CAD build for the part. Positions are in the model's coordinates, mm. Round coordinates to 2 decimals unless told otherwise and drop trailing zeros. Order: outer loops, then holes, each group sorted by start corner. A loop starts at its lowest first (then second) coordinate and runs counter-clockwise, first axis right, second up. Notation, with made-up numbers: M 88.25,77 L 138.25,77 A16 cw 138.25,96 Z; hole C 87,-22 d3. An arc over 180 degrees is marked long. Put each result on its own line as item: value.
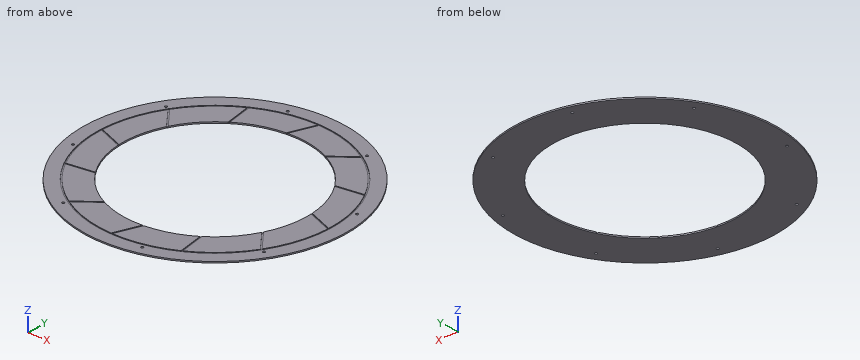
```python
from build123d import *

# Parameters (mm, degrees)
SKETCH1_R                    = 254
SKETCH1_R_2                  = 177.8
BOSS_EXTRUDE1_DEPTH          = 2.54
SKETCH2_R                    = 228.6
SKETCH2_R_2                  = 226.06
CUT_EXTRUDE1_DEPTH           = 1.27
CUT_EXTRUDE2_DEPTH           = 1.27
F_10_0_1935_DIAMETER_HOLE2_D = 4.9149


with BuildPart() as part:
    # Sketch1 → Boss-Extrude1 (new body)
    with BuildSketch(Plane.XY):
        Circle(SKETCH1_R)
        Circle(SKETCH1_R_2, mode=Mode.SUBTRACT)
    extrude(amount=BOSS_EXTRUDE1_DEPTH)

    # Sketch2 → Cut-Extrude1 (cut)
    with BuildSketch(Plane.XY.offset(2.54)):
        Circle(SKETCH2_R)
        Circle(SKETCH2_R_2, mode=Mode.SUBTRACT)
    extrude(amount=-CUT_EXTRUDE1_DEPTH, mode=Mode.SUBTRACT)

    # Sketch4 → Cut-Extrude2 (cut)
    with BuildSketch(Plane.XY.offset(2.54)):
        with BuildLine():
            Line((-226.06, 0), (-176.125415463, -18.479751401))
            Line((-176.125415463, -18.479751401), (-175.243846947, -16.097643731))
            Line((-175.243846947, -16.097643731), (-226.043846947, 2.702379938))
            ThreePointArc((-226.043846947, 2.702379938), (-226.055961701, 1.351214107), (-226.06, 0))
        make_face()
        with BuildLine():
            Line((-195.77370278, 113.03), (-161.768959743, 72.058773562))
            Line((-161.768959743, 72.058773562), (-159.814445179, 73.680955061))
            Line((-159.814445179, 73.680955061), (-194.408523857, 115.36225315))
            ThreePointArc((-194.408523857, 115.36225315), (-195.094598456, 114.198166593), (-195.77370278, 113.03))
        make_face()
        with BuildLine():
            Line((-113.03, 195.77370278), (-104.066641901, 143.289208342))
            Line((-104.066641901, 143.289208342), (-101.562891886, 143.716801448))
            Line((-101.562891886, 143.716801448), (-110.681593797, 197.110903794))
            ThreePointArc((-110.681593797, 197.110903794), (-111.857795108, 196.445812563), (-113.03, 195.77370278))
        make_face()
        with BuildLine():
            Line((0, 226.06), (-18.479751401, 176.125415463))
            Line((-18.479751401, 176.125415463), (-16.097643731, 175.243846947))
            Line((-16.097643731, 175.243846947), (2.702379938, 226.043846947))
            ThreePointArc((2.702379938, 226.043846947), (1.351214107, 226.055961701), (0, 226.06))
        make_face()
        with BuildLine():
            Line((113.03, 195.77370278), (72.058773562, 161.768959743))
            Line((72.058773562, 161.768959743), (73.680955061, 159.814445179))
            Line((73.680955061, 159.814445179), (115.36225315, 194.408523857))
            ThreePointArc((115.36225315, 194.408523857), (114.198166593, 195.094598456), (113.03, 195.77370278))
        make_face()
        with BuildLine():
            Line((195.77370278, 113.03), (143.289208342, 104.066641901))
            Line((143.289208342, 104.066641901), (143.716801448, 101.562891886))
            Line((143.716801448, 101.562891886), (197.110903794, 110.681593797))
            ThreePointArc((197.110903794, 110.681593797), (196.445812563, 111.857795108), (195.77370278, 113.03))
        make_face()
        with BuildLine():
            Line((226.06, 0), (176.125415463, 18.479751401))
            Line((176.125415463, 18.479751401), (175.243846947, 16.097643731))
            Line((175.243846947, 16.097643731), (226.043846947, -2.702379938))
            ThreePointArc((226.043846947, -2.702379938), (226.055961701, -1.351214107), (226.06, 0))
        make_face()
        with BuildLine():
            Line((195.77370278, -113.03), (161.768959743, -72.058773562))
            Line((161.768959743, -72.058773562), (159.814445179, -73.680955061))
            Line((159.814445179, -73.680955061), (194.408523857, -115.36225315))
            ThreePointArc((194.408523857, -115.36225315), (195.094598456, -114.198166593), (195.77370278, -113.03))
        make_face()
        with BuildLine():
            Line((113.03, -195.77370278), (104.066641901, -143.289208342))
            Line((104.066641901, -143.289208342), (101.562891886, -143.716801448))
            Line((101.562891886, -143.716801448), (110.681593797, -197.110903794))
            ThreePointArc((110.681593797, -197.110903794), (111.857795108, -196.445812563), (113.03, -195.77370278))
        make_face()
        with BuildLine():
            Line((0, -226.06), (18.479751401, -176.125415463))
            Line((18.479751401, -176.125415463), (16.097643731, -175.243846947))
            Line((16.097643731, -175.243846947), (-2.702379938, -226.043846947))
            ThreePointArc((-2.702379938, -226.043846947), (-1.351214107, -226.055961701), (0, -226.06))
        make_face()
        with BuildLine():
            Line((-113.03, -195.77370278), (-72.058773562, -161.768959743))
            Line((-72.058773562, -161.768959743), (-73.680955061, -159.814445179))
            Line((-73.680955061, -159.814445179), (-115.36225315, -194.408523857))
            ThreePointArc((-115.36225315, -194.408523857), (-114.198166593, -195.094598456), (-113.03, -195.77370278))
        make_face()
        with BuildLine():
            Line((-195.77370278, -113.03), (-143.289208342, -104.066641901))
            Line((-143.289208342, -104.066641901), (-143.716801448, -101.562891886))
            Line((-143.716801448, -101.562891886), (-197.110903794, -110.681593797))
            ThreePointArc((-197.110903794, -110.681593797), (-196.445812563, -111.857795108), (-195.77370278, -113.03))
        make_face()
    extrude(amount=-CUT_EXTRUDE2_DEPTH, mode=Mode.SUBTRACT)

    # #10 (0.1935) Diameter Hole2 (through all)
    with Locations(Plane.XY.offset(2.54)):
        with Locations((-204.022594751, 117.7925), (-60.97388474, 227.557635786), (117.7925, 204.022594751), (227.557635786, 60.97388474), (204.022594751, -117.7925), (60.97388474, -227.557635786), (-117.7925, -204.022594751), (-227.557635786, -60.97388474)):
            Hole(F_10_0_1935_DIAMETER_HOLE2_D / 2)


solid = part.part
```
Item 1: Pin check, flat tips, straight feed: P1, Ø6.5, axis at x = -204.02, y = 117.79, coming from the -Z side; P2, Ø1.5, axis at y = 25.5, z = 0.5, coming from the +X side; P3, Ø1.5, axis at x = -101, z = 1.5, coming from the +Y side; P4, Ø1.5, axis at x = 162.5, z = 2, coming from the +Y side. Stop position of each tip, or through.
Answers below:
P1: z = 0
P2: x = 252.79
P3: y = 233.38
P4: y = 195.84
Item 2: Band-saw the part on A-A on x = -129. Give the cut face in (y, z).
Answers below:
outline: M -218.8,0 L -122.36,0 L -122.36,2.54 L -185.64,2.54 L -185.64,1.27 L -188.72,1.27 L -188.72,2.54 L -218.8,2.54 Z; M 122.36,0 L 218.8,0 L 218.8,2.54 L 188.72,2.54 L 188.72,1.27 L 185.64,1.27 L 185.64,2.54 L 122.36,2.54 Z
Item 3: Band-saw the part on C-C on y = -187.5. Give the cut face in (x, z).
Answers below:
outline: M -171.35,0 L 171.35,0 L 171.35,2.54 L 130.77,2.54 L 130.77,1.27 L 126.28,1.27 L 126.28,2.54 L 111.62,2.54 L 111.62,1.27 L 109.04,1.27 L 109.04,2.54 L 14.27,2.54 L 14.27,1.27 L 11.56,1.27 L 11.56,2.54 L -103.06,2.54 L -103.06,1.27 L -107.04,1.27 L -107.04,2.54 L -126.28,2.54 L -126.28,1.27 L -130.77,1.27 L -130.77,2.54 L -171.35,2.54 Z
Item 4: Band-saw the part on B-B on y = -45.5. Give the cut face in (x, z), and give its area (3 significant figures).
Answers below:
outline: M -249.89,0 L -171.88,0 L -171.88,2.54 L -221.43,2.54 L -221.43,1.27 L -224.03,1.27 L -224.03,2.54 L -249.89,2.54 Z; M 171.88,0 L 249.89,0 L 249.89,2.54 L 224.03,2.54 L 224.03,1.27 L 221.43,1.27 L 221.43,2.54 L 171.88,2.54 Z
area: 390 mm²
Item 5: Probe line 1 along X through (y, z) = (88, 1.4); line 2 along Y through (x, z) = (138, 1.45); line 3 along Y through (x, z) = (-74, 1.85). List the from-to ranges inside material, lowest first. Write a range as [from, to].
Answers below:
line 1: [-238.27, -210.98], [-208.23, -175], [-171.7, -154.5], [154.5, 208.23], [210.98, 238.27]
line 2: [-213.24, -182.25], [-179.05, -112.11], [112.11, 179.05], [182.25, 213.24]
line 3: [-242.98, -216.29], [-213.61, -163.38], [161.67, 213.61], [216.29, 242.98]
